Geometry: see drawing. Coordinates: mm, zero at the bounding-box minimum. A direction names the side the tool comes from. Coordinates: 2 decimals unless noted, no trailing zeros. Order: outer loops, then holes, each group sorted by start corner. A loop starts at its lowest first (then second) coordinate and runs counter-clockwise, first axis right, second up.
Item 1: Reachability of the marked faces 1 and 2 from +Z, -Z, +X, -X, +Y, -Y: full face, straight path, thin tool, end or side. Return the list, or none.
Item 2: Section A-A on z = 34. Return the cut outline in (x, y), then the cut area to 3 significant figures.
Item 3: Contact query for flat-ended pins moving along their axis: P1, Ø4.5, axis at x = 44.5, z = 34.5, coming from the -Y side (1 decimal); P2, Ø5, axis at x = 9, y = 13.5, coming from the +Z side; P3, Ø7.5, axis at y = 33, z = 31.5, coming from the -X side. Output: stop coordinate, or through.
Item 4: Section B-B on z = 2. Return the cut outline in (x, y), then the cut area to 3 significant figures.
Item 5: Ray query, line 1 (X direction, y = 16, z = 28) (1 decimal); line 2 (Z direction, x = 50, y = 39.5); line 3 (Z direction, x = 59.5, y = 7). Return the intervals inside material, ascending.
Item 6: Mould query, pull axis Y, two halves, no side actions, for the marked faces 3, 4 and 5. Classes: released by +Y, released by -Y, zero draft, split by the parting line, or undercut.
Item 7: Section C-C on z = 25.5. Return the cut outline in (x, y), then the cut area to 3 significant figures.
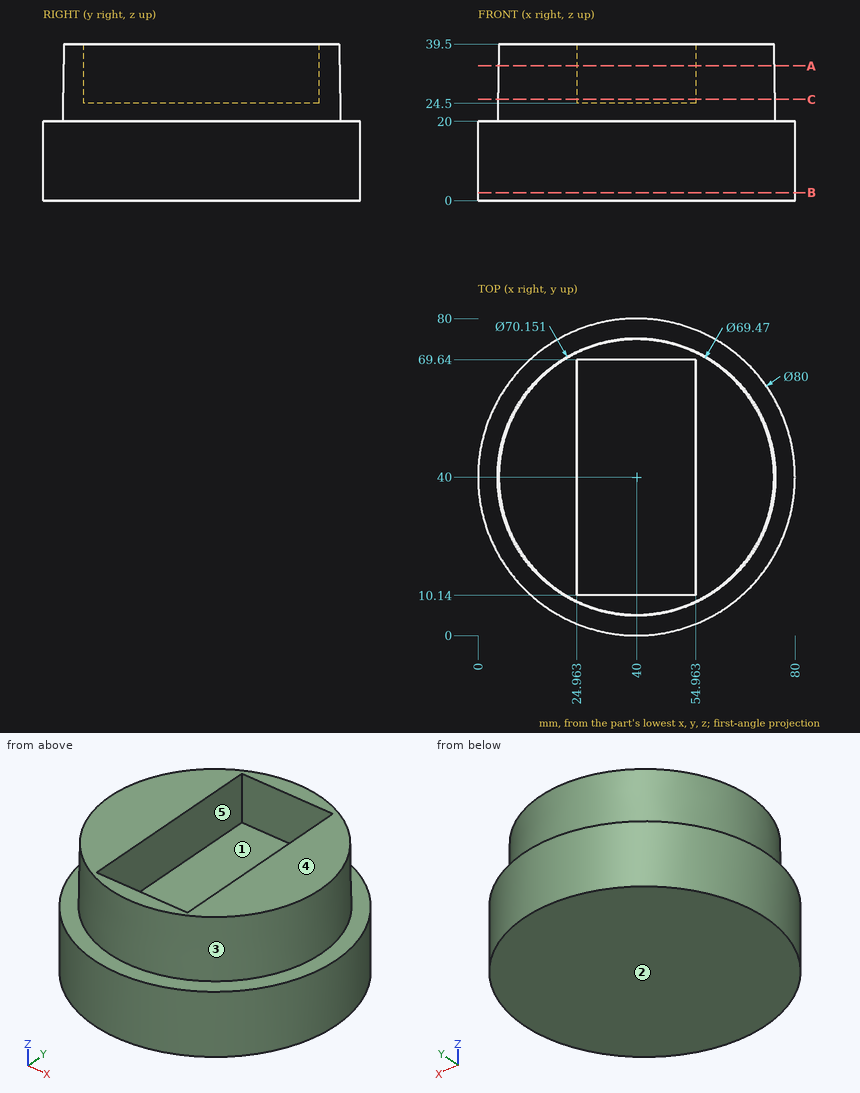
Answer list:
1. face 1: +Z
1. face 2: -Z, +X, -X, +Y, -Y
2. outline: circle Ø69.66 at (40, 40); hole (24.96, 10.14) - (54.96, 10.14) - (54.96, 69.64) - (24.96, 69.64) - close
2. area: 2,030 mm2
3. P1: stops at y = 5.2
3. P2: stops at z = 20
3. P3: stops at x = 5.27
4. outline: circle Ø80 at (40, 40)
4. area: 5,030 mm2
5. line 1: x = 14.6 to 25, 55 to 65.4
5. line 2: z = 0 to 24.5
5. line 3: z = 0 to 20
6. face 3: split by the parting line
6. face 4: zero draft
6. face 5: undercut
7. outline: circle Ø69.96 at (40, 40); hole (24.96, 10.14) - (54.96, 10.14) - (54.96, 69.64) - (24.96, 69.64) - close
7. area: 2,060 mm2
